Geometry: final body of the model. Coordinates: model frame, mm. Face numbers are marked on the shaded views. A direction names the side the tool comes from. Give positions to 0.01 mm unless a question says otherwise; leave off trailing zeros. Write each loop counter-clockwise with the first axis right and the second up, starting at its lowest first coordinate (ties: lowest second). Pieces come first, ordered by that corner, then holes. Notation, with made-up numbers: (71, 57) -> (82, 57) arc R25 ccw to (82, 94) -> close; hole circle Ø2 at (-23.5, -35). An arc over 180 degrees is marked (long way). Answer in a Markdown table with one row per item. Add a question column.
Item 1: Draft query along Z for the marked faces 1, 2 and 3. Return one class per face: +Z half, -Z half, draft (parallel to the pull), parting line (faces both ways), or undercut.
Item 2: Section query A-A on z = 21.25. Output: boundary loops of the cut face in (x, y), plus the area to 3 significant figures.
Item 3: Section query C-C on z = 9.75. Output: boundary loops of the cut face in (x, y), plus the area to 3 significant figures.
Item 4: Material intervals for probe 1 along Z at (x, y) = (4.75, 8); probe 2 along Y at (x, z) = (0, 19); probe 3 along Z at (x, y) = (-1.75, -3.75), sorted ascending. Write a range as from..to.
Item 5: First-contact query: P1, Ø4, axis at x = -2, y = -6, coming from the +Z side; P2, Ø2.5, axis at x = 6.93, y = -4, coming from the -Z side; P3, Ø6, axis at y = 1, z = 6, coming from the -X side; P4, Ø1.5, axis at x = -6.5, z = 3, coming from the -Y side. Flat tips, straight axial feed; report the tip coordinate or a pass-through.
Item 6: Section query B-B on y = -3. State how many separate pieces and enclosed holes the cut face has, plus the area to 3 significant figures.
Item 7: Access query for the marked faces 4 and 5. Directions: +Z, -Z, +X, -X, +Y, -Y. A direction counts if a zero-diameter tool reaches every point of the face in a straight line with its end or side. Return the directions, or none.
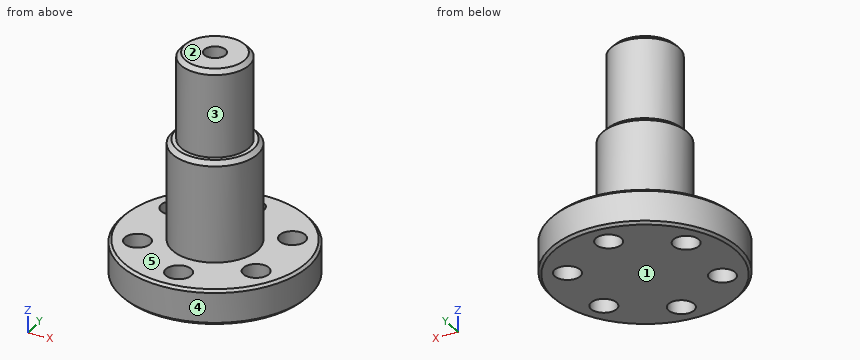
```python
from build123d import *

# Parameters (mm, degrees)
SKETCH_1_R             = 11
SKETCH_1_R_2           = 1.5
EXTRUDE_1_DEPTH        = 4.1
SKETCH_2_R             = 5
EXTRUDE_2_DEPTH        = 22
SKETCH_3_OUTSIDE_W     = 32.122
SKETCH_3_OUTSIDE_H     = 32.122
SKETCH_3_OUTSIDE_R     = 4
CUT_EXTRUDE_1_DEPTH    = 10.2
CHAMFER_1_SIZE         = 0.5
HOLE_WIZARD_M3_1_D     = 2.5
HOLE_WIZARD_M3_1_DEPTH = 9.5
HOLE_WIZARD_M3_1_TIP   = 0.751075774
CHAMFER_2_SIZE         = 0.3


with BuildPart() as part:
    # 草图1 → 凸台-拉伸1 (new body)
    with BuildSketch(Plane.XY):
        Circle(SKETCH_1_R)
        with Locations((0, 8)):
            Circle(SKETCH_1_R_2, mode=Mode.SUBTRACT)
        with Locations((6.92820323, 4)):
            Circle(SKETCH_1_R_2, mode=Mode.SUBTRACT)
        with Locations((6.92820323, -4)):
            Circle(SKETCH_1_R_2, mode=Mode.SUBTRACT)
        with Locations((0, -8)):
            Circle(SKETCH_1_R_2, mode=Mode.SUBTRACT)
        with Locations((-6.92820323, -4)):
            Circle(SKETCH_1_R_2, mode=Mode.SUBTRACT)
        with Locations((-6.92820323, 4)):
            Circle(SKETCH_1_R_2, mode=Mode.SUBTRACT)
    extrude(amount=EXTRUDE_1_DEPTH)

    # 草图2 → 凸台-拉伸2 (add)
    with BuildSketch(Plane.XY.offset(4.1)):
        Circle(SKETCH_2_R)
    extrude(amount=EXTRUDE_2_DEPTH)

    # 草图3 outside → 切除-拉伸1 (cut)
    with BuildSketch(Plane.XY.offset(26.1)):
        Rectangle(SKETCH_3_OUTSIDE_W, SKETCH_3_OUTSIDE_H)
        Circle(SKETCH_3_OUTSIDE_R, mode=Mode.SUBTRACT)
    extrude(amount=-CUT_EXTRUDE_1_DEPTH, mode=Mode.SUBTRACT)

    # 倒角1
    chamfer_1_edges = [part.edges().sort_by_distance(p)[0] for p in [
        (-4, 0, 26.1),
        (-5, 0, 15.9),
    ]]
    chamfer(chamfer_1_edges, length=CHAMFER_1_SIZE)

    # M3 螺纹孔1
    with Locations(Plane.XY.offset(26.1)):
        with Locations((0, 0)):
            Hole(HOLE_WIZARD_M3_1_D / 2, depth=HOLE_WIZARD_M3_1_DEPTH)
            with Locations((0, 0, -(HOLE_WIZARD_M3_1_DEPTH + HOLE_WIZARD_M3_1_TIP / 2))):  # 118° drill point
                Cone(0, HOLE_WIZARD_M3_1_D / 2, HOLE_WIZARD_M3_1_TIP, mode=Mode.SUBTRACT)

    # 倒角2
    chamfer_2_edges = [part.edges().sort_by_distance(p)[0] for p in [
        (-11, 0, 0),
        (-11, 0, 4.1),
    ]]
    chamfer(chamfer_2_edges, length=CHAMFER_2_SIZE)


solid = part.part
```
Findings below:
| question | item | result |
|---|---|---|
| 1 | face 1 | -Z half |
| 1 | face 2 | +Z half |
| 1 | face 3 | draft |
| 2 | outline | circle Ø8 at (0, 0); hole circle Ø2.5 at (0, 0) |
| 2 | area | 45.4 mm^2 |
| 3 | outline | circle Ø10 at (0, 0) |
| 3 | area | 78.5 mm^2 |
| 4 | probe 1 | z = 0..4.1 |
| 4 | probe 2 | y = -4..-1.25, 1.25..4 |
| 4 | probe 3 | z = 0..15.9 |
| 5 | P1 | stops at z = 15.9 |
| 5 | P2 | passes through |
| 5 | P3 | stops at x = -11 |
| 5 | P4 | stops at y = -9.38 |
| 6 | separate pieces | 3 |
| 6 | enclosed holes | 0 |
| 6 | area | 216 mm^2 |
| 7 | face 4 | +Z, -Z |
| 7 | face 5 | +Z |
